The drawing under review shows one solid part. Ordinate dimensions are in mm from its lowest x, y, z. Give positions to 0.01 mm unless a question says otherwise; leave off trailing zeros. Write each loop counter-clockwise with the first axis right and the second up, starting at its lowest first coordinate (ties: lowest second). Pieces come first, ordered by that corner, then holes.
Q1. We need section C-C (y = 1.05). Give the number of separate pieces and of enclosed holes in the cut face, then the cut area to 3 significant figures.
Q2. Insertion check: P1, Ø1.5, axis at x = 69.5, y = 1.5, coming from the +Z side; P2, Ø4, axis at x = 57.15, z = 3.81, coming from the -Y side; P3, Ø2, axis at x = 3.81, z = 57.15, coming from the -Y side; P4, Ø1, axis at x = 71.5, y = 1, coming from the -Z side. Each pin has a flat end and moves straight along its axis. Give the tip position at first contact, or say it passes through.
Q3. We need section A-A (z = 57.15). Write out the cut boundary in (x, y), then the cut area to 3 significant figures.
Q4. For line 1 (X direction, y = 1.7, z = 56); line 2 (X direction, y = 0.45, z = 5) (1 decimal); line 3 (X direction, y = 1.5, z = 44.5), list the stretches that pass through material, from the lowest coordinate up.
Q5. We need section D-D (x = 3.81). Write out the cut boundary in (y, z).
Q6. We need section B-B (x = 57.15). Write out the cut boundary in (y, z), then the cut area to 3 significant figures.
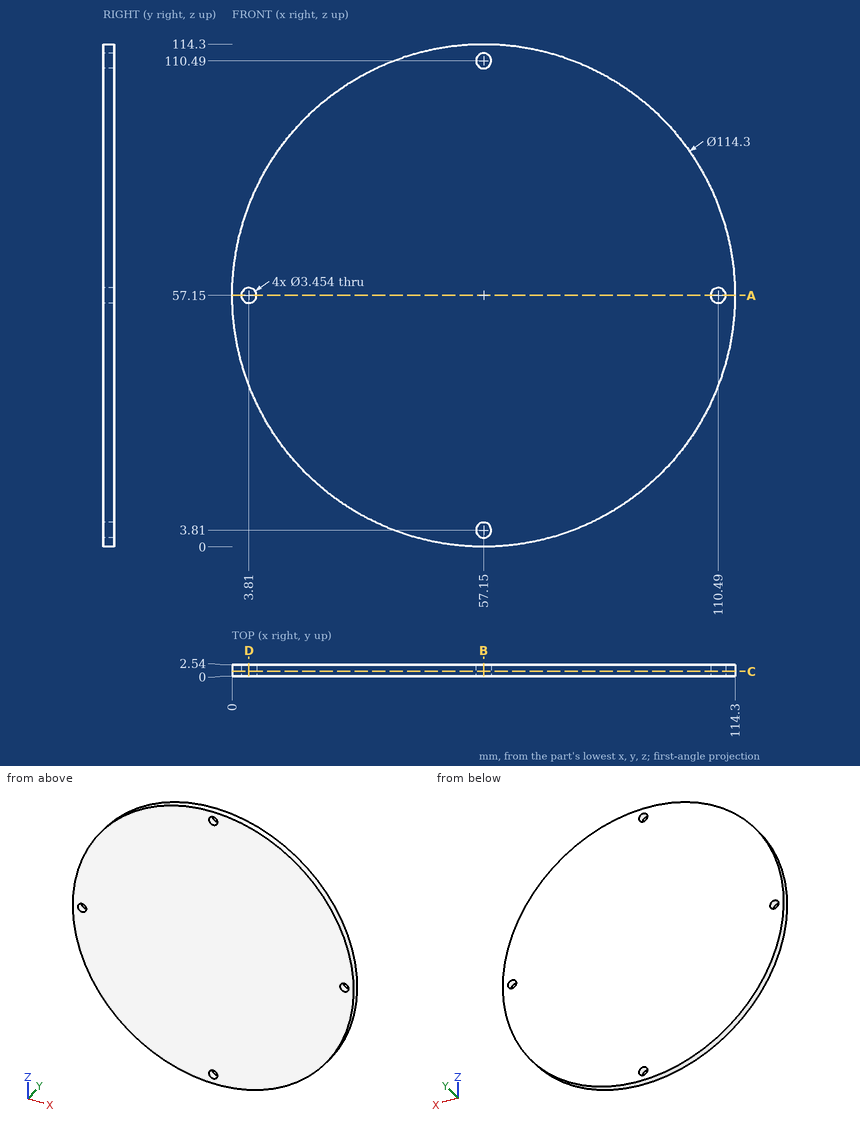
Computed:
1. separate pieces: 1
1. enclosed holes: 4
1. area: 10,200 mm2
2. P1: stops at z = 113.11
2. P2: stops at y = 0
2. P3: passes through
2. P4: stops at z = 1.7
3. outline: (0, 0) - (2.08, 0) - (2.08, 2.54) - (0, 2.54) - close; (5.54, 0) - (108.76, 0) - (108.76, 2.54) - (5.54, 2.54) - close; (112.22, 0) - (114.3, 0) - (114.3, 2.54) - (112.22, 2.54) - close
3. area: 273 mm2
4. line 1: x = 0.01 to 2.52, 5.1 to 109.2, 111.78 to 114.29
4. line 2: x = 33.8 to 55.9, 58.4 to 80.5
4. line 3: x = 1.42 to 112.88
5. outline: (0, 36.63) - (2.54, 36.63) - (2.54, 55.42) - (0, 55.42) - close; (0, 58.88) - (2.54, 58.88) - (2.54, 77.67) - (0, 77.67) - close
6. outline: (0, 0) - (2.54, 0) - (2.54, 2.08) - (0, 2.08) - close; (0, 5.54) - (2.54, 5.54) - (2.54, 108.76) - (0, 108.76) - close; (0, 112.22) - (2.54, 112.22) - (2.54, 114.3) - (0, 114.3) - close
6. area: 273 mm2
